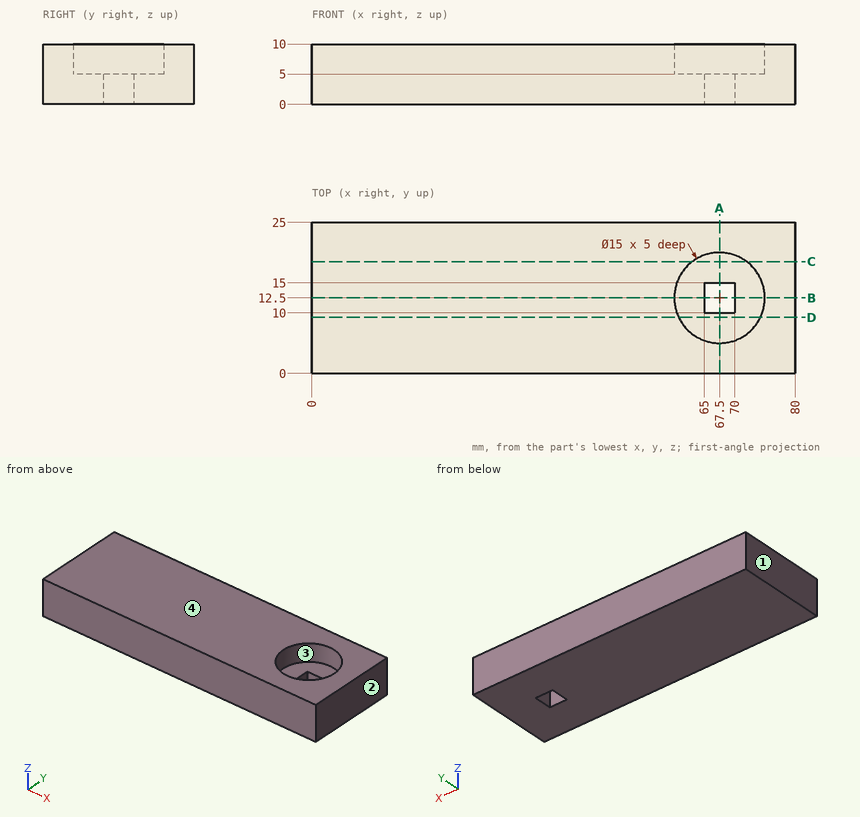
For this review, use the dimensioned drawing (mm, ordinates from the lowest corner) and the shaded views. Coordinates: 2 decimals unless noted, no trailing zeros. Loops run counter-clockwise (first coordinate to the right, second up) from the corner with the lowest first, then second, coordinate; pieces in that order, holes last. Notation, with made-up numbers: M 7.5,45.25 L 30.5,45.25 A38 ccw 30.5,84.25 Z; hole C -17,74 d8. An arc over 180 degrees is marked long. Answer as CSV lines item,"result".
Item 1: For P1, Ø4, axis at x = 49, y = 17, coming from the -Z side, flat-tipped, find the tip position at first contact; note if it passes through.
Answer list:
P1,"z = 0"
Item 2: Add section D-D on y = 9.25. State the section outline as (x, z) points, plus the area to 3 significant figures.
Answer list:
outline,"M 0,0 L 80,0 L 80,10 L 74.26,10 L 74.26,5 L 60.74,5 L 60.74,10 L 0,10 Z"
area,"732 mm²"
Item 3: For probe 1 along Y at (x, z) = (67.5, 8.7); probe 2 along X at (y, z) = (12.25, 1.25); probe 3 along Y at (x, z) = (66, 7.25), list the stretches that pass through material, from the lowest coordinate up.
Answer list:
probe 1,"0 to 5, 20 to 25"
probe 2,"0 to 65, 70 to 80"
probe 3,"0 to 5.15, 19.85 to 25"
Item 4: Add section B-B on y = 12.5. State the section outline as (x, z) points, plus the area to 3 significant figures.
Answer list:
outline,"M 0,0 L 65,0 L 65,5 L 60,5 L 60,10 L 0,10 Z; M 70,0 L 80,0 L 80,10 L 75,10 L 75,5 L 70,5 Z"
area,"700 mm²"
Item 5: The part is to be moulded in two halves that separate along X. For the marked faces 1, 2, 3 and 4, say which applies: pulls with the +X half, pulls with the -X half, needs draft (parallel to the pull), parting line crosses it, or undercut.
Answer list:
face 1,"pulls with the -X half"
face 2,"pulls with the +X half"
face 3,"undercut"
face 4,"needs draft"
Item 6: Add section A-A on x = 67.5. State the section outline as (y, z) points, plus the area to 3 significant figures.
Answer list:
outline,"M 0,0 L 10,0 L 10,5 L 5,5 L 5,10 L 0,10 Z; M 15,0 L 25,0 L 25,10 L 20,10 L 20,5 L 15,5 Z"
area,"150 mm²"
Item 7: Add section C-C on y = 18.5. State the section outline as (x, z) points, plus the area to 3 significant figures.
Answer list:
outline,"M 0,0 L 80,0 L 80,10 L 72,10 L 72,5 L 63,5 L 63,10 L 0,10 Z"
area,"755 mm²"
